from build123d import *

# Parameters (mm, degrees)
BOSS_EXTRUDE1_DEPTH = 3.175
SKETCH2_R           = 2.286
CUT_EXTRUDE1_DEPTH  = 34.89972345
FILLET1_START       = -1
FILLET1_DEPTH       = 5
FILLET1_2_DEPTH     = 3.175
BOSS_EXTRUDE2_DEPTH = 3.175
LPATTERN1_COUNT     = 4
LPATTERN1_PITCH     = 6.35
LPATTERN1_COL_COUNT = 4
LPATTERN1_COL_PITCH = 6.35


with BuildPart() as part:
    # Sketch1 → Boss-Extrude1 (new body)
    with BuildSketch(Plane(origin=(0, 0, 0), x_dir=(1, 0, 0), z_dir=(0, 1, 0))):
        with BuildLine():
            Line((-15.875, 12.7), (-15.875, 17.4625))
            ThreePointArc((-15.875, 17.4625), (-20.6375, 22.225), (-25.4, 17.4625))
            Line((-25.4, 17.4625), (-25.4, -12.7))
            Line((-25.4, -12.7), (15.875, -12.7))
            Line((15.875, -12.7), (15.875, -17.4625))
            ThreePointArc((15.875, -17.4625), (20.6375, -22.225), (25.4, -17.4625))
            Line((25.4, -17.4625), (25.4, 12.7))
            Line((25.4, 12.7), (-15.875, 12.7))
        make_face()
    extrude(amount=BOSS_EXTRUDE1_DEPTH)

    # Sketch2 → Cut-Extrude1 (cut, through all)
    with BuildSketch(Plane(origin=(0, 3.175, 0), x_dir=(1, 0, 0), z_dir=(0, 1, 0))):
        with Locations(Location((-20.6375, 17.4625, 0), (0, 0, 270))):
            Circle(SKETCH2_R)
        with Locations(Location((20.6375, -17.4625, 0), (0, 0, 270))):
            Circle(SKETCH2_R)
    extrude(amount=-CUT_EXTRUDE1_DEPTH, mode=Mode.SUBTRACT)

    # Fillet1: read off the stored shape, not the designer's step
    # Fillet1 outline → Fillet1 (cut)
    with BuildSketch(Plane(origin=(0, 0, 0), x_dir=(1, 0, 0), z_dir=(0, 1, 0)).offset(FILLET1_START)):
        with BuildLine():
            Line((25.4, 12.7), (20.6375, 12.7))
            ThreePointArc((20.6375, 12.7), (24.005096045, 11.305096045), (25.4, 7.9375))
            Line((25.4, 7.9375), (25.4, 12.7))
        make_face()
        with BuildLine():
            Line((-25.4, -12.7), (-20.6375, -12.7))
            ThreePointArc((-20.6375, -12.7), (-24.005096045, -11.305096045), (-25.4, -7.9375))
            Line((-25.4, -7.9375), (-25.4, -12.7))
        make_face()
    extrude(amount=FILLET1_DEPTH, mode=Mode.SUBTRACT)

    # Fillet1 2 outline → Fillet1 2 (add)
    with BuildSketch(Plane(origin=(0, 0, 0), x_dir=(1, 0, 0), z_dir=(0, 1, 0))):
        with BuildLine():
            Line((-15.875, 12.7), (-11.1125, 12.7))
            ThreePointArc((-11.1125, 12.7), (-14.480096045, 14.094903955), (-15.875, 17.4625))
            Line((-15.875, 17.4625), (-15.875, 12.7))
        make_face()
        with BuildLine():
            Line((15.875, -12.7), (11.1125, -12.7))
            ThreePointArc((11.1125, -12.7), (14.480096045, -14.094903955), (15.875, -17.4625))
            Line((15.875, -17.4625), (15.875, -12.7))
        make_face()
    extrude(amount=FILLET1_2_DEPTH)

    # Sketch3 → Boss-Extrude2 (add)
    with BuildSketch(Plane(origin=(0, 3.175, 0), x_dir=(1, 0, 0), z_dir=(0, 1, 0))):
        Polygon((0, 10.16), (2.54, 7.62), (0, 5.08), (2.54, 2.54), (0, 0), (2.54, -2.54), (0, -5.08), (2.54, -7.62), (0, -10.16), (-2.54, -10.16), (0, -7.62), (-2.54, -5.08), (0, -2.54), (-2.54, 0), (0, 2.54), (-2.54, 5.08), (0, 7.62), (-2.54, 10.16), align=None)
    boss_extrude2 = extrude(amount=BOSS_EXTRUDE2_DEPTH)

    # LPattern1: Boss-Extrude2 ×4
    with Locations(*[(-i * LPATTERN1_PITCH, 0, 0) for i in range(1, LPATTERN1_COUNT)]):
        add(boss_extrude2)

    # LPattern1 col: Boss-Extrude2 ×4
    with Locations(*[(i * LPATTERN1_COL_PITCH, 0, 0) for i in range(1, LPATTERN1_COL_COUNT)]):
        add(boss_extrude2)


solid = part.part
Check sheet for the modelled part. Datum: model origin and axes. Units: mm. A direction names the side the tool comes from. Coordinates: 2 decimals unless noted, no trailing zeros. Loops run counter-clockwise (first coordinate to the right, second up) from the corner with the lowest first, then second, coordinate; pieces in that order, holes last. Notation, with made-up numbers: (57.25, -4.5) -> (84.25, -4.5) arc R18 ccw to (84.25, 9.5) -> close; hole circle Ø8 at (44, -31.5). An arc over 180 degrees is marked (long way). Answer in a Markdown table with one row per item.
1. Sectioned sample at A-A, the plane y = 1.75. Record the boundary of the cut face in (x, z) (1 decimal), then the cut area to 3 significant figures.
Check values:
| item | result |
|---|---|
| outline | (-25.4, -17.5) arc R4.8 ccw to (-15.9, -17.5) arc R4.8 cw to (-11.1, -12.7) -> (20.6, -12.7) arc R4.8 ccw to (25.4, -7.9) -> (25.4, 17.5) arc R4.8 ccw to (15.9, 17.5) arc R4.8 cw to (11.1, 12.7) -> (-20.6, 12.7) arc R4.8 ccw to (-25.4, 7.9) -> close; hole circle Ø4.6 at (-20.6, -17.5); hole circle Ø4.6 at (20.6, 17.5) |
| area | 1,420 mm2 |
2. Sectioned sample at B-B, the plane x = 1.5. Record the boundary of the cut face in (y, z) (3 decimals), then the cut area to 3 significant figures.
Check values:
| item | result |
|---|---|
| outline | (0, -12.7) -> (3.175, -12.7) -> (3.175, -8.66) -> (6.35, -8.66) -> (6.35, -6.58) -> (3.175, -6.58) -> (3.175, -3.58) -> (6.35, -3.58) -> (6.35, -1.5) -> (3.175, -1.5) -> (3.175, 1.5) -> (6.35, 1.5) -> (6.35, 3.58) -> (3.175, 3.58) -> (3.175, 6.58) -> (6.35, 6.58) -> (6.35, 8.66) -> (3.175, 8.66) -> (3.175, 12.7) -> (0, 12.7) -> close |
| area | 107 mm2 |
3. Go/stop test with flat-tipped pins: pin 1 (0.8 mm diameter, centred on x = -1, y = 4, fed in from -Z); pin 2 (4 mm diameter, centred on x = 20.64, z = 17.46, fed in from +Y); pin 3 (2 mm diameter, centred on x = -1.5, y = 4, fed in from +Z); pin 4 (2.5 mm diameter, centred on x = 6, y = 1.5, fed in from -Z). Record where each tip stops, or that it passes through.
Check values:
| item | result |
|---|---|
| pin 1 | stops at z = -10.16 |
| pin 2 | passes through |
| pin 3 | stops at z = 12.7 |
| pin 4 | stops at z = -12.7 |
4. Access from +Z, -Z, +X, -X, +Y, -Y to the whole of each face (thin tool, end or side, straight path). Record for faces 1 (the face through (-20, 5, -10.16)), 2 (the face through (-17.76, 4.74, 8.87)), 3 (the face through (-5, 2, 12.7)), 4 (the face through (-7, 6.35, 0)), 5 (the face through (-1.25, 4.74, -3.79)).
Check values:
| item | result |
|---|---|
| face 1 | -Z, +X, -X, +Y |
| face 2 | +Z, +Y |
| face 3 | +Z, -X, +Y, -Y |
| face 4 | +Z, -Z, +X, -X, +Y |
| face 5 | +Y |
5. Material ranges on line 1 along Z through (x, y) = (-20.5, 5.25); line 2 along Z through (x, y) = (11.5, 4.5); line 3 along Y through (x, z) = (23, -10) (3 decimals), recorded low to high. Write a range as [from, to].
Check values:
| item | result |
|---|---|
| line 1 | z = [-10.16, -9.07], [-6.17, -3.99], [-1.09, 1.09], [3.99, 6.17], [9.07, 10.16] |
| line 2 | z = [-10.16, -8.82], [-6.42, -3.74], [-1.34, 1.34], [3.74, 6.42], [8.82, 10.16] |
| line 3 | y = [0, 3.175] |
6. Release check for a two-part mould opening along X. For faces 6 (the face through (-14, 5, 10.16)), 7 (the face through (20.3, 4.74, -8.91)), 8 (the face through (5.06, 4.74, -1.25)) record: released by +X, released by -X, zero draft, split by the parting line, or undercut.
Check values:
| item | result |
|---|---|
| face 6 | zero draft |
| face 7 | released by +X |
| face 8 | undercut |
7. Sectioned sample at D-D, the plane x = 7. Record the boundary of the cut face in (y, z) (3 decimals).
Check values:
| item | result |
|---|---|
| outline | (0, -12.7) -> (3.175, -12.7) -> (3.175, -9.51) -> (6.35, -9.51) -> (6.35, -5.73) -> (3.175, -5.73) -> (3.175, -4.43) -> (6.35, -4.43) -> (6.35, -0.65) -> (3.175, -0.65) -> (3.175, 0.65) -> (6.35, 0.65) -> (6.35, 4.43) -> (3.175, 4.43) -> (3.175, 5.73) -> (6.35, 5.73) -> (6.35, 9.51) -> (3.175, 9.51) -> (3.175, 12.7) -> (0, 12.7) -> close |
